Part model, mm, in its own coordinate system. A direction names the side the tool comes from. Round coordinates to 2 decimals unless told otherwise and drop trailing zeros. Write each loop counter-clockwise with the first axis right and the second up, starting at its lowest first coordinate (ties: lowest second). Pieces come first, ordered by that corner, then holes. Notation, with made-up numbers: M 35.25,89.25 L 50.25,89.25 A23 cw 50.25,100.25 Z; hole C -32,10 d1. An arc over 180 degrees is marked long. Use a Markdown table: item, result. Add a question column.
1) Slice it at D-D on x = -3. Write the cut outline in (y, z), plus the area to 3 significant figures.
2) Wall check: probe 1 along X at (y, z) = (1.25, -16.75); probe 2 along X at (y, z) = (-1.75, -3.25); probe 3 along X at (y, z) = (-4, -12.25). Give the ranges that are in metal, low to high.
3) Which spindle directions (+Z, -Z, +X, -X, +Y, -Y) get a long thin tool onto all of the face, cutting with end or side? Do faces 4 (the face through (-3.8, 0, -11)), 5 (the face through (0, 0, 4)), 6 (the face through (8, 0, -20)). Say none if no direction does.
4) Slice it at A-A on z = -10.75. Write the cut outline in (x, y).
5) Slice it at B-B on z = -17.5. Write the cut outline in (x, y), plus the area to 3 significant figures.
6) Drop flat-ended pins along their axis: P1, Ø1.1, axis at x = -0.5, y = -2.5, coming from the -Z side; P2, Ø4.5, axis at x = -3.5, y = 1, coming from the +Z side; P3, Ø0.5, axis at x = -6.5, y = -3.5, coming from the -Z side; P4, Ø1, axis at x = 2, z = -6.5, coming from the -Y side (3 decimals). Give the stop position or say it passes through.
7) Two-plate mould, pull along X, no slides. Class faces 1 (the face through (-9.4, 0, -7)), 2 (the face through (3.2, 0.14, -0.57)), 3 (the face through (-4, 10, -6)): released by +X, released by -X, zero draft, split by the parting line, or undercut.
Autodesk Inventor part; units mm, degrees
ref_plane "YZ Plane" through (0, 0, 0) normal (1, 0, 0) x (0, 1, 0)
ref_plane "XZ Plane" through (0, 0, 0) normal (0, 1, 0) x (-1, 0, 0)
ref_plane "XY Plane" through (0, 0, 0) normal (0, 0, 1) x (1, 0, 0)
sketch "Schizzo1" plane through (0, 0, 0) normal (0, 0, 1) x (1, 0, 0)
  line L0 (-5.8, 10) -> (5.8, 10)
  line L1 (5.8, 10) -> (5.8, -10)
  line L2 (5.8, -10) -> (-5.8, -10)
  line L3 (-5.8, -10) -> (-5.8, 10)
  line L4 (-5.8, 10) -> (-7.4, 10)
  line L5 (-7.4, 10) -> (-7.4, -10)
  line L6 (-7.4, -10) -> (-5.8, -10)
  line L7 (-5.8, -10) -> (-5.8, 10)
  line L8 (0, 10) -> (0, -10) construction
  line L9 (-7.4, 10) -> (-9.4, 10)
  line L10 (-9.4, 10) -> (-9.4, -10)
  line L11 (-9.4, -10) -> (-7.4, -10)
  line L12 (-7.4, -10) -> (-7.4, 10)
  line L13 (-5.8, 0) -> (5.8, 0) construction
  line L14 (5.8, 10) -> (7.4, 10)
  line L15 (7.4, -10) -> (5.8, -10)
  line L16 (7.4, 10) -> (9.4, 10)
  line L17 (9.4, 10) -> (9.4, -10)
  line L18 (9.4, -10) -> (7.4, -10)
  line L19 (7.4, -10) -> (7.4, 10)
  line L20 (-3.8, -10) -> (-3.8, 10)
  line L21 (3.8, -10) -> (3.8, 10)
  point P0 (0, 0)
  point P1 (0, 0)
  point P2 (-5.8, -10)
  point P3 (-7.4, -10)
  point P4 (5.8, -10)
  point P5 (7.4, -10)
  point P6 (-5.8, -10)
  dimension "d1" = 20
  dimension "d2" = 1.6
  dimension "d3" = 2
  dimension "d6" = 2
  dimension "d7" = 2
  dimension "d20" = 7.6
extrude "Estrusione1" add sketch "Schizzo1" along normal blind 4
extrude "Estrusione2" add sketch "Schizzo1" against normal blind 20 contours L0 L20 L2 L3 | L5 L11 L10 L9 | L0 L1 L2 L21 | L16 L17 L18 L19
extrude "Estrusione3" add sketch "Schizzo1" against normal blind 12 contours L3 L6 L5 L4 | L14 L19 L15 L1
fillet "Raccordo1" radius 2 2 edges at (-3.8, 0, 0) (3.8, 0, 0)
sketch "Schizzo3" plane through (0, 0, 4) normal (0, 0, 1) x (1, 0, 0)
  line L0 (-9.4, 10) -> (-9.4, -10)
  line L1 (-9.4, -10) -> (9.4, -10)
  line L2 (-9.4, 10) -> (-7.4, 10)
  line L3 (-7.4, 10) -> (-7.4, -10)
  line L4 (-7.4, -10) -> (-9.4, -10)
  line L5 (-9.4, -10) -> (-9.4, 10)
  line L6 (9.4, 10) -> (7.4, 10)
  line L7 (7.4, 10) -> (7.4, -10)
  line L8 (7.4, -10) -> (9.4, -10)
  line L9 (9.4, -10) -> (9.4, 10)
  line L10 (9.4, -10) -> (9.4, 10)
  point P0 (0, 0)
  point P1 (9.4, 0)
  dimension "d16" = 2
  dimension "d17" = 2
extrude "Estrusione5" add sketch "Schizzo3" along normal blind 4
fillet "Raccordo3" radius 0.5 4 edges at (7.4, 0, -12) (5.8, 0, -12) (-7.4, 0, -12) (-5.8, 0, -12)
fillet "Raccordo4" radius 2 2 edges at (9.4, 0, 8) (-9.4, 0, 8)
properties part number "Sensore intermedio"
Entries:
| question | item | result |
|---|---|---|
| 1 | outline | M -10,-0.4 L 10,-0.4 L 10,4 L -10,4 Z |
| 1 | area | 88.0 mm^2 |
| 2 | probe 1 | x = -9.4 to -7.4, -5.8 to -3.8, 3.8 to 5.8, 7.4 to 9.4 |
| 2 | probe 2 | x = -9.4 to -3.8, 3.8 to 9.4 |
| 2 | probe 3 | x = -9.4 to -7.33, -5.87 to -3.8, 3.8 to 5.87, 7.33 to 9.4 |
| 3 | face 4 | -Z, +Y, -Y |
| 3 | face 5 | +Z, +Y, -Y |
| 3 | face 6 | -Z, +X, -X, +Y, -Y |
| 4 | outline | M -9.4,-10 L -3.8,-10 L -3.8,10 L -9.4,10 Z; M 3.8,-10 L 9.4,-10 L 9.4,10 L 3.8,10 Z |
| 5 | outline | M -9.4,-10 L -7.4,-10 L -7.4,10 L -9.4,10 Z; M -5.8,-10 L -3.8,-10 L -3.8,10 L -5.8,10 Z; M 3.8,-10 L 5.8,-10 L 5.8,10 L 3.8,10 Z; M 7.4,-10 L 9.4,-10 L 9.4,10 L 7.4,10 Z |
| 5 | area | 160 mm^2 |
| 6 | P1 | stops at z = 0 |
| 6 | P2 | stops at z = 4 |
| 6 | P3 | stops at z = -12 |
| 6 | P4 | passes through |
| 7 | face 1 | released by -X |
| 7 | face 2 | undercut |
| 7 | face 3 | zero draft |
